from build123d import *

# Parameters (mm, degrees)
ESQUISSE1_W        = 19
ESQUISSE1_H        = 12
BOSS_EXTRU_1_DEPTH = 10
ESQUISSE2_W        = 20
ESQUISSE2_H        = 15
BOSS_EXTRU_2_DEPTH = 2
ESQUISSE3_W        = 1
ESQUISSE3_H        = 5
BOSS_EXTRU_3_DEPTH = 8


with BuildPart() as part:
    # Esquisse1 → Boss.-Extru.1 (new body)
    with BuildSketch(Plane(origin=(0, 0, 0), x_dir=(1, 0, 0), z_dir=(0, 1, 0))):
        with Locations((9.5, 6)):
            Rectangle(ESQUISSE1_W, ESQUISSE1_H)
    extrude(amount=BOSS_EXTRU_1_DEPTH)

    # Esquisse2 → Boss.-Extru.2 (add)
    with BuildSketch(Plane.XY):
        with Locations((9.5, 5)):
            Rectangle(ESQUISSE2_W, ESQUISSE2_H)
    extrude(amount=BOSS_EXTRU_2_DEPTH)

    # Esquisse3 → Boss.-Extru.3 (add)
    with BuildSketch(Plane(origin=(0, 0, -12), x_dir=(-1, 0, 0), z_dir=(0, 0, -1))):
        with Locations((-9.5, 5)):
            Rectangle(ESQUISSE3_W, ESQUISSE3_H)
        with Locations((-2, 5)):
            Rectangle(ESQUISSE3_W, ESQUISSE3_H)
    extrude(amount=BOSS_EXTRU_3_DEPTH)


solid = part.part
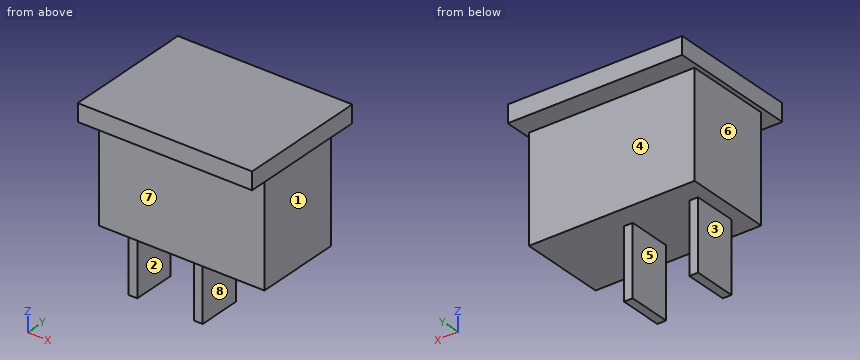
Can you work these out from the model? Positions are in its coordinate system, mm. Face numbers are marked on the shaded views. A direction names the side the tool comes from. Coordinates: 2 decimals unless noted, no trailing zeros. Write each loop counter-clockwise with the first axis right and the second up, starting at its lowest first coordinate (ties: lowest second). Pieces come first, ordered by that corner, then holes. Notation, with made-up numbers: (30.5, 25.5) - (56.5, 25.5) arc R12 ccw to (56.5, 40.5) - close; hole circle Ø2 at (1, 15.25). An arc over 180 degrees is marked (long way). Return JSON: item names as keys, results as strings. Group by question number.
Item 1: If we section it at C-C (y = 4): Write out the boundary of the cut face in (x, z).
Item 2: I'm going to push flat-ended pins straight in: pin 1 Ø3 at (y, z) = (3.5, -4) entering from -X; pin 2 Ø4 at (x, y) = (6.5, 0.5) entering from -Z; pin 3 Ø4 at (y, z) = (4, -16.5) entering from +X. Where does each tip first touch, or does it pass through?
Item 3: If we section it at A-A (z = -14.25): Write out the boundary of the cut face in (x, y).
Item 4: Please list where these lines run through material, in increasing order: probe 1 along Y at (x, z) = (7, -9.5); probe 2 along Z at (x, y) = (11.75, 1); probe 3 along Z at (x, y) = (11.5, 11.75).
Item 5: If we section it at B-B (x = 13): Write out the boundary of the cut face in (y, z).
Item 6: Which directions (+Z, -Z, +X, -X, +Y, -Y) give clear straight access to the entire face, cutting with the end or side of a thin tool? Please do the marked faces 4, 5, 6, 7 and 8.
Item 7: If we section it at D-D (z = -10.25): Write out the boundary of the cut face in (x, y).
Item 8: We'd pull the mould along X, two halves only. Please class the marked faces 1, 2 and 3: pulls with the +X half, pulls with the -X half, needs draft (parallel to the pull), parting line crosses it, or undercut.
Return value:
{
 "1": {"outline": "(-0.5, 0) - (0, 0) - (0, -12) - (1.5, -12) - (1.5, -20) - (2.5, -20) - (2.5, -12) - (9, -12) - (9, -20) - (10, -20) - (10, -12) - (19, -12) - (19, 0) - (19.5, 0) - (19.5, 2) - (-0.5, 2) - close"},
 "2": {"pin 1": "stops at x = 0", "pin 2": "stops at z = -12", "pin 3": "stops at x = 10"},
 "3": {"outline": "(1.5, 2.5) - (2.5, 2.5) - (2.5, 7.5) - (1.5, 7.5) - close; (9, 2.5) - (10, 2.5) - (10, 7.5) - (9, 7.5) - close"},
 "4": {"probe 1": "y = 0 to 10", "probe 2": "z = -12 to 2", "probe 3": "z = 0 to 2"},
 "5": {"outline": "(-2.5, 0) - (0, 0) - (0, -12) - (10, -12) - (10, 0) - (12.5, 0) - (12.5, 2) - (-2.5, 2) - close"},
 "6": {"face 4": "-Z, +X, -X, +Y", "face 5": "-Z, +Y, -Y", "face 6": "-Z, -X, +Y, -Y", "face 7": "-Z, +X, -X, -Y", "face 8": "-Z, +X, +Y, -Y"},
 "7": {"outline": "(0, 0) - (19, 0) - (19, 10) - (0, 10) - close"},
 "8": {"face 1": "pulls with the +X half", "face 2": "undercut", "face 3": "pulls with the -X half"}
}
